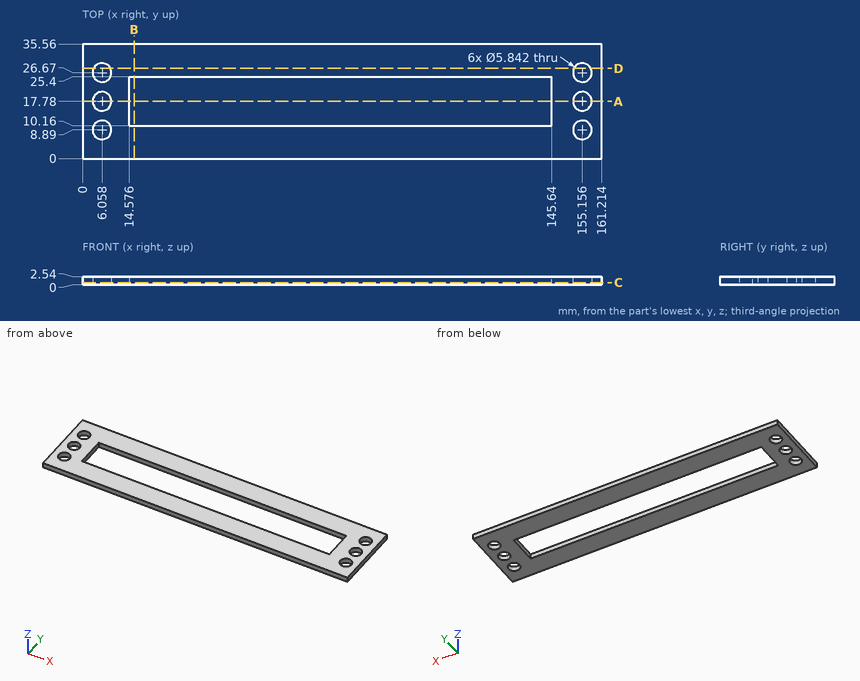
Geometry: see drawing. Coordinates: mm, zero at the bounding-box minimum. Coordinates: 2 decimals unless noted, no trailing zeros. Order: outer loops, then holes, each group sorted by start corner. A loop starts at its lowest first (then second) coordinate and runs counter-clockwise, first axis right, second up. Notation, with made-up numbers: M 65,22 L 118,22 A9 ccw 118,26 Z; hole C 23.25,39 d2. An arc over 180 degrees is marked long. Write item = value, one per line. Start each with the question number.
(1) Section C-C on z = 0.65. Output: boundary loops of the cut face in (x, y).
(2) First-contact query: P1, Ø4.5, axis at x = 6.06, y = 17.78, coming from the +Z side; P2, Ø0.8, axis at x = 84.5, z = 1.5, coming from the -Y side. Flat tips, straight axial feed; report the tip coordinate or a pass-through.
(3) Line query: line 1 along Y through (x, z) = (135.5, 0.35); line 2 along X through (y, z) = (29, 2.4) (1 decimal); line 3 along X through (y, z) = (10, 1) (1 decimal). Output: solid intervals per line, ascending. Write a range as [from, to].
(4) Section A-A on y = 17.78. Output: boundary loops of the cut face in (x, z) (1 decimal).
(5) Section B-B on x = 16. Output: boundary loops of the cut face in (y, z).
(6) Section D-D on y = 28. Output: boundary loops of the cut face in (x, z) (1 decimal).
Result set:
q1.outline = M 0,0 L 161.21,0 L 161.21,35.56 L 0,35.56 Z; hole C 6.06,8.89 d5.84; hole C 6.06,17.78 d5.84; hole C 6.06,26.67 d5.84; hole M 14.58,10.16 L 145.64,10.16 L 145.64,25.4 L 14.58,25.4 Z; hole C 155.16,8.89 d5.84; hole C 155.16,17.78 d5.84; hole C 155.16,26.67 d5.84
q2.P1 = through
q2.P2 = 0
q3.line_1 = [0, 10.16], [25.4, 35.56]
q3.line_2 = [0, 4.3], [7.8, 153.4], [156.9, 161.2]
q3.line_3 = [0, 3.4], [8.8, 152.5], [157.9, 161.2]
q4.outline = M 0,0 L 3.1,0 L 3.1,2.5 L 0,2.5 Z; M 9,0 L 14.6,0 L 14.6,2.5 L 9,2.5 Z; M 145.6,0 L 152.2,0 L 152.2,2.5 L 145.6,2.5 Z; M 158.1,0 L 161.2,0 L 161.2,2.5 L 158.1,2.5 Z
q5.outline = M 0,0 L 10.16,0 L 10.16,2.54 L 0,2.54 Z; M 25.4,0 L 35.56,0 L 35.56,2.54 L 25.4,2.54 Z
q6.outline = M 0,0 L 3.5,0 L 3.5,2.5 L 0,2.5 Z; M 8.7,0 L 152.6,0 L 152.6,2.5 L 8.7,2.5 Z; M 157.8,0 L 161.2,0 L 161.2,2.5 L 157.8,2.5 Z
